Geometry check sheet. Reference: the model listing, model coordinates, mm. A direction names the side the tool comes from. Coordinates: 2 decimals unless noted, no trailing zeros. Write each loop counter-clockwise with the first axis right and the second up, starting at its lowest first coordinate (ties: lowest second). Pieces come first, ordered by that corner, then holes. Notation, with made-up numbers: M 29,-11.5 L 36,-11.5 A24 ccw 36,9.5 Z; hole C 2,52 d2. An arc over 180 degrees is marked long. Write item = value, one per line. Start each with the question number.
Autodesk Inventor part; units mm, degrees
ref_plane "YZ Plane" through (0, 0, 0) normal (1, 0, 0) x (0, 1, 0)
ref_plane "XZ Plane" through (0, 0, 0) normal (0, 1, 0) x (-1, 0, 0)
ref_plane "XY Plane" through (0, 0, 0) normal (0, 0, 1) x (1, 0, 0)
sketch "Sketch1" plane through (0, 0, 0) normal (1, 0, 0) x (0, 1, 0)
  circle A0 centre (0, 0) radius 75
  dimension "d0" = 150
extrude "Extrusion1" add sketch "Sketch1" along normal blind 200
sketch "Sketch2" plane through (200, 0, 0) normal (1, 0, 0) x (0, 0, -1)
  circle A0 centre (0, 0) radius 67.5
  dimension "d3" = 135
extrude "Extrusion2" cut sketch "Sketch2" against normal blind 180
sketch "Sketch3" plane through (200, 0, 0) normal (1, 0, 0) x (0, 0, -1)
  circle A0 centre (0, 0) radius 67.5
  circle A1 centre (0, 0) radius 80
  dimension "d6" = 160
extrude "Extrusion3" add sketch "Sketch3" along normal blind 10 contours A0 | A1
sketch "Sketch4" plane through (210, 0, 0) normal (1, 0, 0) x (0, 0, -1)
  circle A0 centre (0, 0) radius 20
  dimension "d9" = 40
extrude "Extrusion4" add sketch "Sketch4" along normal blind 20
sketch "Sketch5" plane through (230, 0, 0) normal (1, 0, 0) x (0, 0, -1)
  circle A0 centre (0, 0) radius 12.5
  dimension "d12" = 25
extrude "Extrusion5" cut sketch "Sketch5" against normal blind 40
equation "\"BendRadius\" = Thickness"
equation "\"BendReliefWidth\" = Thickness"
equation "\"BendReliefDepth\" = 0.5 * Thickness"
equation "\"CornerReliefSize\" = 4 * Thickness"
equation "\"MinimumRemnant\" = 2 * Thickness"
equation "\"TransitionRadius\" = BendRadius"
equation "\"JacobiRadiusSize\" = BendRadius"
equation "\"GapSize\" = Thickness"
properties part number "Container1"
Q1. Set-up check for faces 4 (the face through (98.6, -9.764, -74.362)), 5 (the face through (230, 9, -9)), 6 (the face through (20, 1, 1)), 7 (the face through (210, -17, -17)): record each of +Z, -Z, +X, -X, +Y, -Y from which the full face is reachable in a straight line by a thin tool's end or side.
Q2. Cross-section at A-A on y = 0. Enter the section's corners in (x, z), and give its area (3 significant figures).
Q3. Draft check along Z on faces 1 (the face through (204.93, 78.1, 17.34)), 2 (the face through (0, -1, 1)), 3 (the face through (200, -14, 1)). Enter one of: pulls with the +Z half, pulls with the -Z half, needs draft (parallel to the pull), parting line crosses it, or undercut.
Q4. Scan lines: L1, parallel to Y at x = 206.5, z = 0; L2, parallel to Y at x = 69, z = 2; L3, parallel to X at y = -33.5, z = -27.5. Record each from-to range of solid material in increasing order.
Q5. Cross-section at C-C on z = -37. Enter the section's corners in (x, y), and give its area (3 significant figures).
Q6. Gauge pin test, flat ends, axial feed: pin 1 (1.5 mm diameter, centred on x = 205.5, y = 53, fed in from +Z); pin 2 (8 mm diameter, centred on x = 173.5, y = 38.5, fed in from +Z); pin 3 (1.5 mm diameter, centred on x = 70, z = 10.5, fed in from +Y); pin 4 (4 mm diameter, centred on y = -31.5, z = 52, fed in from -X). Record the tip position at first contact, or that the pin passes through.
Q7. Cross-section at D-D on x = 216. Enter the section's corners in (y, z), and give its area (3 significant figures).
Values found:
q1.face_4 = -X
q1.face_5 = +Z, -Z, +X, +Y, -Y
q1.face_6 = none
q1.face_7 = +X
q2.outline = M 0,-75 L 200,-75 L 200,-80 L 210,-80 L 210,-20 L 230,-20 L 230,-12.5 L 200,-12.5 L 200,-67.5 L 20,-67.5 L 20,67.5 L 200,67.5 L 200,12.5 L 230,12.5 L 230,20 L 210,20 L 210,80 L 200,80 L 200,75 L 0,75 Z
q2.area = 7,350 mm²
q3.face_1 = parting line crosses it
q3.face_2 = needs draft
q3.face_3 = undercut
q4.L1 = -80 to -12.5, 12.5 to 80
q4.L2 = -74.97 to -67.47, 67.47 to 74.97
q4.L3 = 0 to 20, 200 to 210
q5.outline = M 0,-65.24 L 200,-65.24 L 200,-70.93 L 210,-70.93 L 210,70.93 L 200,70.93 L 200,65.24 L 0,65.24 Z; hole M 20,-56.46 L 200,-56.46 L 200,56.46 L 20,56.46 Z
q5.area = 7,190 mm²
q6.pin_1 = 60.58
q6.pin_2 = 66.59
q6.pin_3 = 74.36
q6.pin_4 = 0
q7.outline = C 0,0 d40; hole C 0,0 d25
q7.area = 766 mm²
